```python
from build123d import *

# Parameters (mm, degrees)
SKETCH1_R           = 11.8745
BOSS_EXTRUDE1_DEPTH = 23.876
SKETCH2_R           = 9.398
BOSS_EXTRUDE2_DEPTH = 3.3401
SKETCH3_R           = 2.9972
BOSS_EXTRUDE3_DEPTH = 1.524
SKETCH4_R           = 0.9906
BOSS_EXTRUDE4_DEPTH = 6.731
SKETCH5_R           = 4.2926
BOSS_EXTRUDE5_DEPTH = 2.032
CUT_EXTRUDE1_DEPTH  = 2.032
SKETCH7_W           = 0.381
SKETCH7_H           = 3.048
BOSS_EXTRUDE6_DEPTH = 4.572
FILLET1_R           = 1.27
FILLET2_R           = 0.254


with BuildPart() as part:
    # Sketch1 → Boss-Extrude1 (new body)
    with BuildSketch(Plane(origin=(0, 0, 0), x_dir=(1, 0, 0), z_dir=(0, 1, 0))):
        Circle(SKETCH1_R)
    extrude(amount=BOSS_EXTRUDE1_DEPTH)

    # Sketch2 → Boss-Extrude2 (add)
    with BuildSketch(Plane(origin=(0, 23.876, 0), x_dir=(1, 0, 0), z_dir=(0, 1, 0))):
        Circle(SKETCH2_R)
    extrude(amount=BOSS_EXTRUDE2_DEPTH)

    # Sketch3 → Boss-Extrude3 (add)
    with BuildSketch(Plane(origin=(0, 27.2161, 0), x_dir=(1, 0, 0), z_dir=(0, 1, 0))):
        Circle(SKETCH3_R)
    extrude(amount=BOSS_EXTRUDE3_DEPTH)

    # Sketch4 → Boss-Extrude4 (add)
    with BuildSketch(Plane(origin=(0, 28.7401, 0), x_dir=(1, 0, 0), z_dir=(0, 1, 0))):
        Circle(SKETCH4_R)
    extrude(amount=BOSS_EXTRUDE4_DEPTH)

    # Sketch5 → Boss-Extrude5 (add)
    with BuildSketch(Plane.XZ):
        Circle(SKETCH5_R)
    extrude(amount=BOSS_EXTRUDE5_DEPTH)

    # Sketch6 → Cut-Extrude1 (cut)
    with BuildSketch(Plane.XZ.offset(2.032)):
        with BuildLine():
            Line((2.16198617, 3.7084), (-2.16198617, 3.7084))
            ThreePointArc((-2.16198617, 3.7084), (0, 4.2926), (2.16198617, 3.7084))
        make_face()
    extrude(amount=-CUT_EXTRUDE1_DEPTH, mode=Mode.SUBTRACT)

    # Sketch7 → Boss-Extrude6 (add)
    with BuildSketch(Plane.XZ):
        with Locations((-8.89, 0)):
            Rectangle(SKETCH7_W, SKETCH7_H)
        with Locations((8.89, 0)):
            Rectangle(SKETCH7_W, SKETCH7_H)
    extrude(amount=BOSS_EXTRUDE6_DEPTH)

    # Fillet1
    fillet1_edges = [part.edges().sort_by_distance(p)[0] for p in [
        (-11.8745, 0, 0),
        (-9.398, 23.876, 0),
        (-9.398, 27.2161, 0),
    ]]
    fillet(fillet1_edges, radius=FILLET1_R)

    # Fillet2
    fillet2_edges = [part.edges().sort_by_distance(p)[0] for p in [
        (-0.9906, 35.4711, 0),
    ]]
    fillet(fillet2_edges, radius=FILLET2_R)


solid = part.part
```
For this review, take the finished solid that the model builds, in its own axes (mm). A direction names the side the tool comes from. Coordinates: 2 decimals unless noted, no trailing zeros. Order: outer loops, then holes, each group sorted by start corner. A loop starts at its lowest first (then second) coordinate and runs counter-clockwise, first axis right, second up. Notation, with made-up numbers: (38.25, 19.5) -> (69.25, 19.5) arc R23 cw to (69.25, 28.5) -> close; hole circle Ø11 at (73, -25). An arc over 180 degrees is marked (long way). Answer as CSV lines item,"result".
Q1. Draft analysis for pull direction X (two halves, no side actions). For faces 1 (the face through (-1.22, 25.54, -9.32)), 2 (the face through (3.5, 27.216, -0.1)), 3 (the face through (-8.7, -2, 0)), state which applies: released by +X, released by -X, zero draft, split by the parting line, or undercut.
Model answer:
face 1,"split by the parting line"
face 2,"zero draft"
face 3,"undercut"
Q2. Wall thickness on line 1 along Y through (x, z) = (0.25, -2.5); line 2 along Y through (x, z) = (6.5, 0); line 3 along X through (y, z) = (20, -7.25): over which ranges is each line inside the solid? List them lowest first. Write a range as [from, to].
Model answer:
line 1,"y = [-2.03, 28.74]"
line 2,"y = [0, 27.22]"
line 3,"x = [-9.4, 9.4]"
Q3. We need section A-A (x = 0). State the section outline as (y, z) points.
Model answer:
outline,"(-2.03, -4.29) -> (0, -4.29) -> (0, -10.6) arc R1.27 ccw to (1.27, -11.87) -> (23.88, -11.87) -> (23.88, -10.67) arc R1.27 cw to (25.15, -9.4) -> (25.95, -9.4) arc R1.27 ccw to (27.22, -8.13) -> (27.22, -3) -> (28.74, -3) -> (28.74, -0.99) -> (35.22, -0.99) arc R0.25 ccw to (35.47, -0.74) -> (35.47, 0.74) arc R0.25 ccw to (35.22, 0.99) -> (28.74, 0.99) -> (28.74, 3) -> (27.22, 3) -> (27.22, 8.13) arc R1.27 ccw to (25.95, 9.4) -> (25.15, 9.4) arc R1.27 cw to (23.88, 10.67) -> (23.88, 11.87) -> (1.27, 11.87) arc R1.27 ccw to (0, 10.6) -> (0, 3.71) -> (-2.03, 3.71) -> close"
Q4. Clearance check with flat-ended pins moving along their axes: pin 1 Ø5 at (y, z) = (22.5, -3) entering from -X; pin 2 Ø2 at (x, y) = (-1.5, 25.5) entering from -Z; pin 3 Ø6 at (y, z) = (17, -5.5) entering from -X. State where each tip first meets the part, or that it passes through.
Model answer:
pin 1,"stops at x = -11.86"
pin 2,"stops at z = -9.47"
pin 3,"stops at x = -11.61"
Q5. We need section B-B (y = 9). State the section outline as (x, z) points, plus the area to 3 significant figures.
Model answer:
outline,"circle Ø23.75 at (0, 0)"
area,"443 mm2"
Q6. For faces 4 (the face through (-9.08, -2, 0)), 5 (the face through (0, -1, 3.708)), 6 (the face through (8.7, -2, 0)), 7 (the face through (-1, 28.74, -1)), 8 (the face through (9.08, -2, 0)), list the 3-axis set-ups (+Z, -Z, +X, -X, +Y, -Y) from which the entire face can be reached by the end or side of a thin tool; tool diameter is ignored.
Model answer:
face 4,"+Z, -Z, -X, -Y"
face 5,"+Z, +X, -X, -Y"
face 6,"+Z, -Z, -Y"
face 7,"+Y"
face 8,"+Z, -Z, +X, -Y"
